Check sheet for the modelled part. Datum: model origin and axes. Units: mm. A direction names the side the tool comes from. Round coordinates to 2 decimals unless told otherwise and drop trailing zeros. Write each loop counter-clockwise with the first axis right and the second up, starting at its lowest first coordinate (ties: lowest second). Pieces come first, ordered by that corner, then holes. Notation, with made-up numbers: (53, -17) -> (110, -17) arc R17 cw to (110, 6) -> close; hole circle Ø6 at (34, 18.25). An arc over 180 degrees is marked (long way). One line per item, written item: value.
Autodesk Inventor part; units mm, degrees
ref_plane "YZ Plane" through (0, 0, 0) normal (1, 0, 0) x (0, 1, 0)
ref_plane "XZ Plane" through (0, 0, 0) normal (0, 1, 0) x (-1, 0, 0)
ref_plane "XY Plane" through (0, 0, 0) normal (0, 0, 1) x (1, 0, 0)
sketch "Sketch1" plane through (0, 0, 0) normal (0, 0, 1) x (1, 0, 0)
  line L0 (-11.658, 3.4387) -> (-11.658, -21.9613)
  line L1 (-11.658, 3.4387) -> (108.992, 3.4387)
  line L2 (108.992, 3.4387) -> (108.992, -21.9613)
  line L3 (108.992, -21.9613) -> (-11.658, -21.9613)
  point P0 (0, 0)
  dimension "d0" = 25.4
  dimension "d1" = 120.65
  dimension "d2" = 25.4
extrude "Extrusion1" add sketch "Sketch1" along normal blind 6.35
ref_plane "Work Plane1" through (-11.658, -21.9613, 6.35) normal (0, 1, 0) x (1, 0, 0)
sketch "Sketch3" plane through (-11.658, -21.9613, 6.35) normal (0, 1, 0) x (1, 0, 0)
  line L0 (0, 0) -> (120.65, 0)
  line L1 (120.65, -25.4) -> (0, -25.4)
  line L2 (120.65, 0) -> (120.65, -25.4)
  line L3 (0, -25.4) -> (12.7, -25.4)
  line L4 (12.7, -25.4) -> (12.7, 0)
  line L5 (12.7, 0) -> (19.05, 0)
  line L6 (19.05, 0) -> (19.05, -25.4)
  line L7 (19.05, -25.4) -> (12.7, -25.4)
  line L8 (19.05, -25.4) -> (63.5, -25.4)
  line L9 (63.5, -25.4) -> (63.5, 0)
  line L10 (63.5, 0) -> (69.85, 0)
  line L11 (69.85, 0) -> (69.85, -25.4)
  line L12 (69.85, -25.4) -> (63.5, -25.4)
  line L13 (69.85, -25.4) -> (114.3, -25.4)
  line L14 (114.3, -25.4) -> (114.3, 0)
  line L15 (120.65, 0) -> (114.3, 0)
  line L16 (120.65, 0) -> (120.65, -25.4)
  line L17 (114.3, -25.4) -> (120.65, -25.4)
  point P0 (11.658, 6.35)
  dimension "d8" = 12.7
  dimension "d9" = 6.35
  dimension "d10" = 25.4
  dimension "d11" = 44.45
  dimension "d12" = 6.35
  dimension "d13" = 25.4
  dimension "d14" = 44.45
extrude "Extrusion3" add sketch "Sketch3" along normal blind 25.4 contours L0 L6 L1 L4 | L0 L11 L1 L9 | L0 L2 L1 L14
ref_plane "Work Plane2" through (7.392, -21.9613, 31.75) normal (1, 0, 0) x (0, 0, -1)
sketch "Sketch4" plane through (7.392, -21.9613, 31.75) normal (1, 0, 0) x (0, 0, -1)
  line L0 (25.4, 0) -> (0, 0)
  line L1 (25.4, 25.4) -> (25.4, 0)
  line L2 (0, 25.4) -> (25.4, 25.4)
  line L3 (0, 0) -> (0, 25.4)
  point P0 (31.75, 21.9613)
sketch "Sketch5" plane through (108.992, -21.9613, 0) normal (1, 0, 0) x (0, 0, -1)
  line L0 (-31.75, 0) -> (-31.75, 31.75)
  line L1 (-31.75, 31.75) -> (-31.75, 12.7)
  line L2 (-31.75, 12.7) -> (-19.05, 12.7)
  circle A0 centre (-19.05, 12.7) radius 3.175
  point P0 (0, 21.9613)
  dimension "d17" = 19.05
  dimension "d18" = 12.7
  dimension "d19" = 6.35
extrude "Extrusion4" cut sketch "Sketch5" against normal blind 76.2
sketch "Sketch6" plane through (-11.658, -21.9613, 0) normal (0, -1, 0) x (1, 0, 0)
  line L0 (114.3, 6.35) -> (114.3, 31.75)
  line L1 (69.85, 6.35) -> (114.3, 6.35)
  line L2 (63.5, 6.35) -> (63.5, 31.75)
  line L3 (19.05, 6.35) -> (63.5, 6.35)
  line L4 (19.05, 31.75) -> (19.05, 6.35)
  line L5 (19.05, 6.35) -> (19.05, 16.51)
  line L6 (19.05, 6.35) -> (29.21, 6.35)
  line L7 (29.21, 6.35) -> (19.05, 16.51)
  line L8 (63.5, 6.35) -> (53.34, 6.35)
  line L9 (53.34, 6.35) -> (63.5, 16.51)
  line L10 (63.5, 6.35) -> (63.5, 16.51)
  line L11 (114.3, 6.35) -> (104.14, 6.35)
  line L12 (104.14, 6.35) -> (114.3, 16.51)
  line L13 (114.3, 6.35) -> (114.3, 16.51)
  point P0 (11.658, 0)
  dimension "d22" = 10.16
  dimension "d23" = 10.16
  dimension "d24" = 10.16
  dimension "d25" = 10.16
extrude "Extrusion5" add sketch "Sketch6" against normal blind 5.08
sketch "Sketch7" plane through (-11.658, 3.4387, 0) normal (0, 1, 0) x (1, 0, 0)
  line L0 (19.05, -31.75) -> (19.05, -6.35)
  line L1 (63.5, -6.35) -> (19.05, -6.35)
  line L2 (63.5, -6.35) -> (63.5, -31.75)
  line L3 (19.05, -6.35) -> (19.05, -16.51)
  line L4 (19.05, -6.35) -> (29.21, -6.35)
  line L5 (29.21, -6.35) -> (19.05, -16.51)
  line L6 (63.5, -6.35) -> (53.34, -6.35)
  line L7 (53.34, -6.35) -> (63.5, -16.51)
  line L8 (63.5, -6.35) -> (63.5, -16.51)
  line L9 (114.3, -6.35) -> (104.14, -6.35)
  line L10 (104.14, -6.35) -> (114.3, -16.51)
  line L11 (114.3, -6.35) -> (114.3, -16.51)
  point P0 (11.658, 0)
  dimension "d28" = 10.16
  dimension "d29" = 10.16
  dimension "d30" = 10.16
  dimension "d31" = 10.16
extrude "Extrusion6" add sketch "Sketch7" against normal blind 5.08
properties part number "side"
Item 1: Sectioned sample at D-D on x = 66.5. Enter the section's corners in (y, z).
Answer:
outline: (-21.96, 0) -> (3.44, 0) -> (3.44, 6.35) -> (-21.96, 6.35) -> close
Item 2: Mould release check, pull along Y, two halves, no side actions. Record for faces 4 (the flat face through (49, -16.881, 9)), 5 (the flat face through (97.49, -19.46, 11.36)), 6 (the flat face through (53, 3.439, 9)): pulls with the +Y half, pulls with the -Y half, needs draft (parallel to the pull), parting line crosses it, or undercut.
Answer:
face 4: undercut
face 5: needs draft
face 6: pulls with the +Y half
Item 3: Sectioned sample at B-B on z = 19.05. Enter the section's corners in (x, y), and give its area (3 significant figures).
Answer:
outline: (1.04, -21.96) -> (7.39, -21.96) -> (7.39, 3.44) -> (1.04, 3.44) -> close; (51.84, -21.96) -> (58.19, -21.96) -> (58.19, -12.44) -> (51.84, -12.44) -> close; (51.84, -6.09) -> (58.19, -6.09) -> (58.19, 3.44) -> (51.84, 3.44) -> close; (102.64, -21.96) -> (108.99, -21.96) -> (108.99, -12.44) -> (102.64, -12.44) -> close; (102.64, -6.09) -> (108.99, -6.09) -> (108.99, 3.44) -> (102.64, 3.44) -> close
area: 403 mm^2
Item 4: Tool access check on faces 1 (the flat face through (97.49, 0.93, 11.36)), 2 (the flat face through (7.392, -9, 22)), 3 (the flat face through (-5, -9, 6.35)). Record the directions out of +Z, -Z, +X, -X, +Y, -Y that give a thin tool (end or side, any length) a straight path to the whole face; none if there is none.
Answer:
face 1: +Z, +Y, -Y
face 2: +Z
face 3: +Z, -X, +Y, -Y
Item 5: Sectioned sample at A-A on z = 27. Enter the section's corners in (x, y).
Answer:
outline: (1.04, -21.96) -> (7.39, -21.96) -> (7.39, 3.44) -> (1.04, 3.44) -> close; (51.84, -21.96) -> (58.19, -21.96) -> (58.19, 3.44) -> (51.84, 3.44) -> close; (102.64, -21.96) -> (108.99, -21.96) -> (108.99, 3.44) -> (102.64, 3.44) -> close
Item 6: Depth check by flat-ended pin: P1, Ø10, axis at x = 24.5, y = -4, coming from the +Z side; P2, Ø12.5, axis at y = -9.5, z = 23, coming from the -X side. Enter the tip coordinate at first touch or a pass-through.
Answer:
P1: stops at z = 6.35
P2: stops at x = 1.04
Item 7: Thickness scan on line 1 (X direction, y = -15.25, z = 9); line 2 (Y direction, x = 57.25, z = 19.05); line 3 (Y direction, x = 102.5, z = 12). Record the ranges inside material, lowest first.
Answer:
line 1: x = 1.04 to 7.39, 51.84 to 58.19, 102.64 to 108.99
line 2: y = -21.96 to -12.44, -6.09 to 3.44
line 3: y = -21.96 to -16.88, -1.64 to 3.44
Item 8: Sectioned sample at C-C on y = -7.25. Enter the section's corners in (x, z).
Answer:
outline: (-11.66, 0) -> (108.99, 0) -> (108.99, 16.59) -> (102.64, 16.59) -> (102.64, 6.35) -> (58.19, 6.35) -> (58.19, 16.59) -> (51.84, 16.59) -> (51.84, 6.35) -> (7.39, 6.35) -> (7.39, 31.75) -> (1.04, 31.75) -> (1.04, 6.35) -> (-11.66, 6.35) -> close; (51.84, 21.51) -> (58.19, 21.51) -> (58.19, 31.75) -> (51.84, 31.75) -> close; (102.64, 21.51) -> (108.99, 21.51) -> (108.99, 31.75) -> (102.64, 31.75) -> close
